from build123d import *

# Parameters (mm, degrees)
F0_W     = 19.05
F0_H     = 19.05
F1_DEPTH = 6.35
F3_DEPTH = 3.81
F5_DEPTH = 6.35
F7_DEPTH = 3.048
F8_R     = 1.905
F9_DEPTH = 3.303


with BuildPart() as f1:
    # F0 (on Top) → F1 (new body)
    with BuildSketch(Plane.XY):
        Rectangle(F0_W, F0_H)
    extrude(amount=-F1_DEPTH)

    # F2 (on face) → F3 (join)
    with BuildSketch(Plane.XY):
        with BuildLine():
            ThreePointArc((6.35, 0), (0, -6.35), (-6.35, 0))
            Line((-6.35, 0), (-6.35, 9.525))
            Line((-6.35, 9.525), (-9.525, 9.525))
            Line((-9.525, 9.525), (-9.525, -9.525))
            Line((-9.525, -9.525), (9.525, -9.525))
            Line((9.525, -9.525), (9.525, 9.525))
            Line((9.525, 9.525), (6.35, 9.525))
            Line((6.35, 9.525), (6.35, 0))
        make_face()
    extrude(amount=F3_DEPTH)

    # F4 (on face) → F5 (join)
    with BuildSketch(Plane.XY.offset(3.81)):
        with BuildLine():
            Line((-3.175, 9.525), (-9.525, 9.525))
            Line((-9.525, 9.525), (-9.525, -9.525))
            Line((-9.525, -9.525), (9.525, -9.525))
            Line((9.525, -9.525), (9.525, 9.525))
            Line((9.525, 9.525), (3.175, 9.525))
            Line((3.175, 9.525), (3.175, 0))
            ThreePointArc((3.175, 0), (0, -3.175), (-3.175, 0))
            Line((-3.175, 0), (-3.175, 9.525))
        make_face()
    extrude(amount=F5_DEPTH)

    # F6 (on face) → F7 (cut)
    with BuildSketch(Plane.XY):
        Polygon((2.383013, -4.1275), (4.766026, 0), (2.383013, 4.1275), (-2.383013, 4.1275), (-4.766026, 0), (-2.383013, -4.1275), align=None)
    extrude(amount=-F7_DEPTH, mode=Mode.SUBTRACT)

    # F8 (on face) → F9 (cut, through all)
    with BuildSketch(Plane.XY.offset(-3.048)):
        Circle(F8_R)
    extrude(amount=-F9_DEPTH, mode=Mode.SUBTRACT)


solid = f1.part
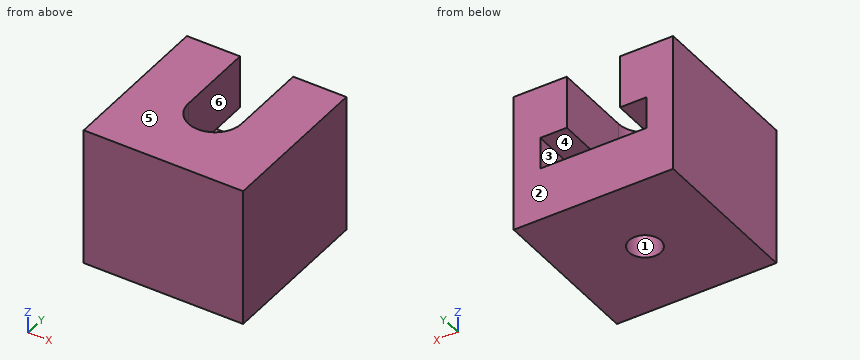
Work out the finished part from the listing and answer in its coordinate system (mm). Face numbers are marked on the shaded views. A direction names the side the tool comes from. Coordinates: 2 decimals unless noted, no trailing zeros. Write each loop counter-clockwise with the first axis right and the second up, starting at its lowest first coordinate (ties: lowest second). Pieces come first, ordered by that corner, then holes. Notation, with made-up numbers: (59.5, 33) - (99.5, 33) arc R7 cw to (99.5, 39) - close; hole circle Ø8 at (50.25, 34.25). An arc over 180 degrees is marked (long way). One line per question, with ' | ' between items.
1) For the marked faces 4, 5 and 6, determine the directions among +Z, -Z, +X, -X, +Y, -Y from which every point of the face is accessible in a straight line to the end or side of a thin tool.
Checks:
face 4: +Y | face 5: +Z, +X, -X, +Y, -Y | face 6: +Z, +Y
2) Find section C-C, the plane y = 7.5. Determine the outline of the cut face in (x, z) (3 decimals).
Checks:
outline: (-9.525, -6.35) - (9.525, -6.35) - (9.525, 10.16) - (3.175, 10.16) - (3.175, 3.81) - (6.35, 3.81) - (6.35, 0) - (-6.35, 0) - (-6.35, 3.81) - (-3.175, 3.81) - (-3.175, 10.16) - (-9.525, 10.16) - close
3) A flat-ended cylindrical pin translates along its axis: P1, Ø4, axis at x = -1, y = 1, coming from the +Z side. Find the tip coordinate at first contact, or state that the pin passes through.
Checks:
P1: z = -3.05
4) Find section B-B, the plane z = 9. Determine the outline of the cut face in (x, y) (3 decimals).
Checks:
outline: (-9.525, -9.525) - (9.525, -9.525) - (9.525, 9.525) - (3.175, 9.525) - (3.175, 0) arc R3.175 cw to (-3.175, 0) - (-3.175, 9.525) - (-9.525, 9.525) - close
5) Find section D-D, the plane y = -6. Determine the outline of the cut face in (x, z) (3 decimals), and give its area (3 significant figures).
Checks:
outline: (-9.525, -6.35) - (9.525, -6.35) - (9.525, 10.16) - (-9.525, 10.16) - close; hole (-2.079, 0) - (2.079, 0) - (2.079, 3.81) - (-2.079, 3.81) - close | area: 299 mm2
6) Consider probe 1 along Z at (x, y) = (-4.5, -4); probe 2 along X at (y, z) = (1.25, 5.5) (3 decimals); probe 3 along Y at (x, z) = (0, -4.3) (3 decimals). Determine where each line is inside the solid, lowest interval first. Write a range as [from, to].
Checks:
probe 1: [-6.35, 0], [3.81, 10.16] | probe 2: [-9.525, -3.175], [3.175, 9.525] | probe 3: [-9.525, -1.905], [1.905, 9.525]
7) The mould has two halves that part along Y. Classify the marked faces 1, 2 and 3: +Y half, -Y half, draft (parallel to the pull), parting line (faces both ways), or undercut.
Checks:
face 1: undercut | face 2: +Y half | face 3: draft
